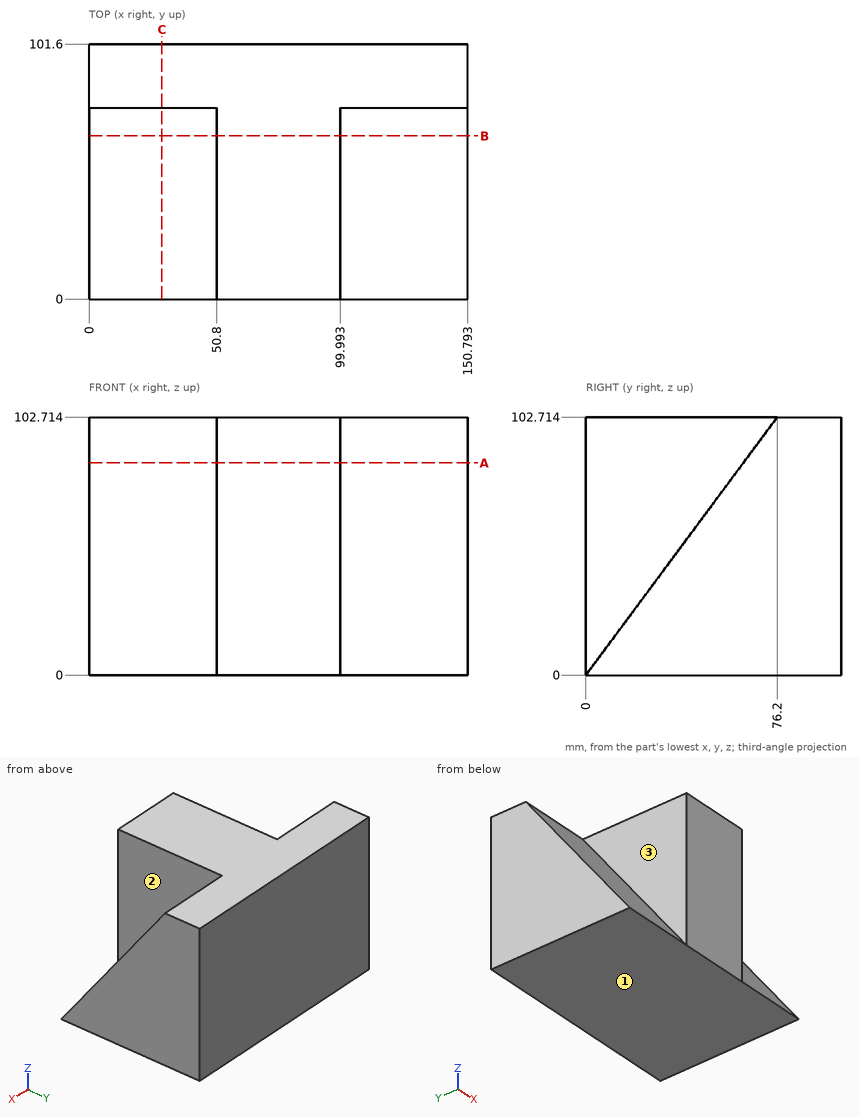
Part print with two shaded views. Sizes in mm from the minimum x, y, z corner. A direction names the side the tool comes from. Coordinates: 2 decimals unless noted, no trailing zeros. Order: outer loops, then holes, each group sorted by start corner. A loop starts at its lowest first (then second) coordinate and runs counter-clockwise, first axis right, second up. Notation, with made-up numbers: (49.5, 43.5) - (73.5, 43.5) arc R15 cw to (73.5, 50.5) - close; hole circle Ø6 at (49.25, 34.5). An arc over 180 degrees is marked (long way). Answer in a Markdown table with one row per item.
1. 3-axis set-ups, long thin cutter, end or side, ignore diameter. For the marked faces 1, 2 and 3: which of +Z, -Z, +X, -X, +Y, -Y reach the whole face in a straight line?
Answer:
| item | result |
|---|---|
| face 1 | -Z, +X, -X, +Y, -Y |
| face 2 | +Z, +X, -Y |
| face 3 | +Z, -X, -Y |
2. Slice it at C-C, the plane x = 29. List the corners of the cut face in (y, z), then the cut area to 3 significant figures.
Answer:
| item | result |
|---|---|
| outline | (0, 0) - (101.6, 0) - (101.6, 102.71) - (76.2, 102.71) - close |
| area | 6,520 mm² |
3. Slice it at B-B, the plane y = 65. List the corners of the cut face in (x, z), then the cut area to 3 significant figures.
Answer:
| item | result |
|---|---|
| outline | (0, 0) - (150.79, 0) - (150.79, 87.62) - (99.99, 87.62) - (99.99, 102.71) - (50.8, 102.71) - (50.8, 87.62) - (0, 87.62) - close |
| area | 14,000 mm² |
4. Flat gauge pins, fed straight in: P1, Ø1.5, axis at x = 131.5, z = 30.5, coming from the -Y side; P2, Ø1, axis at x = 20.5, z = 77, coming from the -Y side; P3, Ø8, axis at x = 48.5, y = 16, coming from the -Z side; P4, Ø8, axis at x = 132, z = 87.5, coming from the -Y side. Where does each tip first touch, or does it go through?
Answer:
| item | result |
|---|---|
| P1 | y = 22.07 |
| P2 | y = 56.75 |
| P3 | z = 0 |
| P4 | y = 61.95 |
5. Drill centre lines: L1, parallel to X at y = 42.5, z = 74; L2, parallel to Y at x = 120.5, z = 13 (1 decimal); L3, parallel to Y at x = 36.5, z = 58.5. Where is each one in solid material? Low to high. Write a range as from..to.
Answer:
| item | result |
|---|---|
| L1 | 50.8..99.99 |
| L2 | 9.6..101.6 |
| L3 | 43.4..101.6 |
6. Slice it at A-A, the plane z = 84.5. List the corners of the cut face in (x, y), then the cut area to 3 significant figures.
Answer:
| item | result |
|---|---|
| outline | (0, 62.69) - (50.8, 62.69) - (50.8, 0) - (99.99, 0) - (99.99, 62.69) - (150.79, 62.69) - (150.79, 101.6) - (0, 101.6) - close |
| area | 8,950 mm² |
